```python
from build123d import *

# Parameters (mm, degrees)
SKETCH1_R           = 16
SKETCH1_R_2         = 1.5
SKETCH1_R_3         = 5
BOSS_EXTRUDE1_DEPTH = 4
SKETCH2_R           = 8
SKETCH2_R_2         = 5
BOSS_EXTRUDE2_DEPTH = 15


with BuildPart() as part:
    # Sketch1 → Boss-Extrude1 (new body)
    with BuildSketch(Plane(origin=(0, 0, 0), x_dir=(1, 0, 0), z_dir=(0, 1, 0))):
        Circle(SKETCH1_R)
        with Locations((8.27314934, -8.27314934)):
            Circle(SKETCH1_R_2, mode=Mode.SUBTRACT)
        Circle(SKETCH1_R_3, mode=Mode.SUBTRACT)
        with Locations((-8.27314934, -8.27314934)):
            Circle(SKETCH1_R_2, mode=Mode.SUBTRACT)
        with Locations((8.27314934, 8.27314934)):
            Circle(SKETCH1_R_2, mode=Mode.SUBTRACT)
        with Locations((-8.27314934, 8.27314934)):
            Circle(SKETCH1_R_2, mode=Mode.SUBTRACT)
    extrude(amount=BOSS_EXTRUDE1_DEPTH)

    # Sketch2 → Boss-Extrude2 (add)
    with BuildSketch(Plane(origin=(0, 4, 0), x_dir=(1, 0, 0), z_dir=(0, 1, 0))):
        Circle(SKETCH2_R)
        Circle(SKETCH2_R_2, mode=Mode.SUBTRACT)
    extrude(amount=BOSS_EXTRUDE2_DEPTH)


solid = part.part
```
Model file for the job. Use its own axes, mm. A direction names the side the tool comes from. Give positions to 0.01 mm unless a question says otherwise; leave off trailing zeros. Order: outer loops, then holes, each group sorted by start corner. A loop starts at its lowest first (then second) coordinate and runs counter-clockwise, first axis right, second up.
1) Saw through at C-C, the plane x = 8.5. Write the cut outline in (y, z), then the cut area to 3 significant figures.
2) 3-axis set-ups, long thin cutter, end or side, ignore diameter. For faces 1 (the cylindrical face through (-1.73, 11.4, 7.81)), 2 (the cylindrical face through (-1.08, 9.37, 4.88)): which of +Z, -Z, +X, -X, +Y, -Y reach the whole face in a straight line?
3) Saw through at A-A, the plane z = 0. Write the cut outline in (x, y).
4) Saw through at D-D, the plane y = 6.5. Write the cut outline in (x, z), then the cut area to 3 significant figures.
5) Wall check: probe 1 along Z at (x, y) = (0, 6.25); probe 2 along Z at (x, y) = (7, 3.25). Give the ranges that are in metal, low to high.
6) Saw through at B-B, the plane x = 0. Write the cut outline in (y, z).
7) Mould opens along X. For faces 3 (the flat face through (-3.8, 4, -7.3)), 4 (the cylindrical face through (9.704, 1.972, 7.823)), 5 (the cylindrical face through (-3.47, 1.97, 15.62)) say: +X half, -X half, draft (parallel to the pull), parting line (faces both ways), or undercut.
8) Pin check, flat tips, straight feed: pin 1 (3 mm diameter, centred on x = 12, z = 8.5, fed in from -Y); pin 2 (4 mm diameter, centred on x = 5.5, y = 11.5, fed in from -Z); pin 3 (8 mm diameter, centred on y = 5, z = -7, fed in from +X); pin 4 (4 mm diameter, centred on y = 15.5, z = -0.5, fed in from -X). Stop position of each tip, or through.
Computed:
1. outline: (0, -13.56) - (4, -13.56) - (4, -9.76) - (0, -9.76) - close; (0, -6.79) - (4, -6.79) - (4, 6.79) - (0, 6.79) - close; (0, 9.76) - (4, 9.76) - (4, 13.56) - (0, 13.56) - close
1. area: 84.7 mm2
2. face 1: +Y
2. face 2: +Y, -Y
3. outline: (-16, 0) - (-5, 0) - (-5, 19) - (-8, 19) - (-8, 4) - (-16, 4) - close; (5, 0) - (16, 0) - (16, 4) - (8, 4) - (8, 19) - (5, 19) - close
4. outline: circle Ø16 at (0, 0); hole circle Ø10 at (0, 0)
4. area: 123 mm2
5. probe 1: z = -8 to -5, 5 to 8
5. probe 2: z = -14.39 to -9.07, -7.48 to 7.48, 9.07 to 14.39
6. outline: (0, -16) - (4, -16) - (4, -8) - (19, -8) - (19, -5) - (0, -5) - close; (0, 5) - (19, 5) - (19, 8) - (4, 8) - (4, 16) - (0, 16) - close
7. face 3: draft
7. face 4: undercut
7. face 5: parting line
8. pin 1: stops at y = 0
8. pin 2: stops at z = -7.19
8. pin 3: stops at x = 15.69
8. pin 4: stops at x = -8
